Geometry check sheet. Reference: the model listing, model coordinates, mm. Face numbers are marked on the shaded views. Give positions to 0.01 mm unless a question says otherwise; leave off trailing zeros. Loops run counter-clockwise (first coordinate to the right, second up) from the corner with the lowest first, then second, coordinate; pieces in that order, holes last. Notation, with made-up numbers: (8, 1.5) - (42, 1.5) arc R25 cw to (42, 32.5) - close; hole circle Ø11 at (-2, -18.75). An arc over 180 degrees is marked (long way). One line per question, with ' | ' between items. Start each with the question number.
from build123d import *

# Parameters (mm, degrees)
SKETCH1_R             = 5
BOSS_EXTRUDE1_DEPTH   = 24
BOSS_EXTRUDE1_2_DEPTH = 24
BOSS_EXTRUDE1_3_DEPTH = 24
BOSS_EXTRUDE1_4_DEPTH = 24
BOSS_EXTRUDE3_START   = 2
SKETCH1_5_W           = 56.57
SKETCH1_5_H           = 40
SKETCH1_5_R           = 5
BOSS_EXTRUDE3_DEPTH   = 2


with BuildPart() as part:
    # Sketch1 → Boss-Extrude1 (new body)
    with BuildSketch(Plane(origin=(0, 0, 0), x_dir=(1, 0, 0), z_dir=(0, 1, 0))):
        with Locations(Location((-28.285, 5, 0), (0, 0, 270))):
            Circle(SKETCH1_R)
    extrude(amount=-BOSS_EXTRUDE1_DEPTH)



with BuildPart() as body_2:
    # Sketch1 → Boss-Extrude1 2 (new body)
    with BuildSketch(Plane(origin=(0, 0, 0), x_dir=(1, 0, 0), z_dir=(0, 1, 0))):
        with Locations(Location((-28.285, 61.57, 0), (0, 0, 270))):
            Circle(SKETCH1_R)
    extrude(amount=-BOSS_EXTRUDE1_2_DEPTH)


with BuildPart() as body_3:
    # Sketch1 → Boss-Extrude1 3 (new body)
    with BuildSketch(Plane(origin=(0, 0, 0), x_dir=(1, 0, 0), z_dir=(0, 1, 0))):
        with Locations(Location((28.285, 61.57, 0), (0, 0, 270))):
            Circle(SKETCH1_R)
    extrude(amount=-BOSS_EXTRUDE1_3_DEPTH)


with BuildPart() as body_4:
    # Sketch1 → Boss-Extrude1 4 (new body)
    with BuildSketch(Plane(origin=(0, 0, 0), x_dir=(1, 0, 0), z_dir=(0, 1, 0))):
        with Locations(Location((28.285, 5, 0), (0, 0, 270))):
            Circle(SKETCH1_R)
    extrude(amount=-BOSS_EXTRUDE1_4_DEPTH)


with BuildPart() as part_1:
    add(part.part)

    add(body_2.part)  # Boss-Extrude3 merges body 2

    add(body_3.part)  # Boss-Extrude3 merges body 3

    add(body_4.part)  # Boss-Extrude3 merges body 4
    # Sketch1_5 → Boss-Extrude3 (add)
    with BuildSketch(Plane(origin=(0, 0, 0), x_dir=(1, 0, 0), z_dir=(0, 1, 0)).offset(BOSS_EXTRUDE3_START)):
        with BuildLine():
            ThreePointArc((15, 33.285), (0, 18.285), (-15, 33.285))
            Line((-15, 33.285), (-15, 66.57))
            Line((-15, 66.57), (-28.285, 66.57))
            ThreePointArc((-28.285, 66.57), (-24.749466094, 65.105533906), (-23.285, 61.57))
            ThreePointArc((-23.285, 61.57), (-28.285, 56.57), (-33.285, 61.57))
            Line((-33.285, 61.57), (-33.285, 5))
            ThreePointArc((-33.285, 5), (-28.285, 10), (-23.285, 5))
            ThreePointArc((-23.285, 5), (-24.749466094, 1.464466094), (-28.285, 0))
            Line((-28.285, 0), (28.285, 0))
            ThreePointArc((28.285, 0), (24.749466094, 8.535533906), (33.285, 5))
            Line((33.285, 5), (33.285, 61.57))
            ThreePointArc((33.285, 61.57), (24.749466094, 58.034466094), (28.285, 66.57))
            Line((28.285, 66.57), (15, 66.57))
            Line((15, 66.57), (15, 33.285))
        make_face()
        with Locations((0, -20)):
            Rectangle(SKETCH1_5_W, SKETCH1_5_H)
        with Locations(Location((-28.285, 61.57, 0), (0, 0, 90))):
            Circle(SKETCH1_5_R)
        with Locations(Location((28.285, 61.57, 0), (0, 0, 90))):
            Circle(SKETCH1_5_R)
        with Locations(Location((28.285, 5, 0), (0, 0, 270))):
            Circle(SKETCH1_5_R)
        with Locations(Location((-28.285, 5, 0), (0, 0, 270))):
            Circle(SKETCH1_5_R)
    extrude(amount=-BOSS_EXTRUDE3_DEPTH)


solid = part_1.part
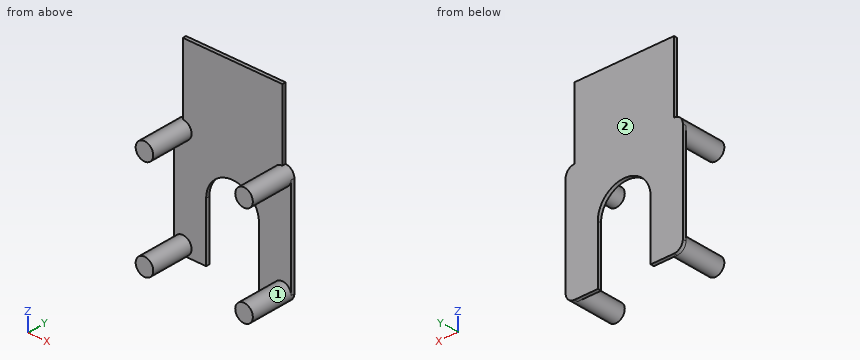
(1) Mould release check, pull along Z, two halves, no side actions. Record for the marked faces 1 and 2: pulls with the +Z half, pulls with the -Z half, needs draft (parallel to the pull), parting line crosses it, or undercut.
(2) Material ranges on line 1 (X direction, y = -15.5, z = -5) (3 decimals); line 2 (Z direction, x = -28, y = -15); line 3 (Y direction, x = 6, z = -4.5), recorded low to high.
(3) Section check C-C, the plane x = -26. Record the boundary of the cut face in (y, z).
(4) Section check A-A, the plane y = -7.5. Record the boundary of the cut face in (x, z) (3 decimals).
(5) Section check B-B, the plane z = -25. Record the boundary of the cut face in (x, y) (3 decimals), and give its area (3 significant figures).
(6) Section check D-D, the plane z = 20. Record the boundary of the cut face in (x, y) (3 decimals).
(7) Depth check by flat-ended pin: pin 1 Ø8 at (x, y) = (12.5, -4.5) entering from -Z; pin 2 Ø3 at (x, z) = (-13, -1.5) entering from -Y; pin 3 Ø1.6 at (y, z) = (1, 15) entering from -X (3 decimals); pin 4 Ø1.6 at (y, z) = (0.5, 10) entering from +X (3 decimals). Enter the tip coordinate at first touch or a pass-through.
Numbers:
1) face 1: undercut | face 2: needs draft
2) line 1: -33.285 to -23.285, 23.285 to 33.285 | line 2: -66.56 to -56.58, -9.99 to -0.01 | line 3: 0 to 2
3) outline: (-24, -66.02) - (0, -66.02) - (0, -66.57) - (2, -66.57) - (2, 40) - (0, 40) - (0, -0.55) - (-24, -0.55) - (-24, -9.45) - (0, -9.45) - (0, -57.12) - (-24, -57.12) - close
4) outline: circle Ø10 at (-28.285, -61.57); circle Ø10 at (-28.285, -5); circle Ø10 at (28.285, -61.57); circle Ø10 at (28.285, -5)
5) outline: (-33.285, 0) - (-12.504, 0) - (-12.504, 2) - (-33.285, 2) - close; (12.504, 0) - (33.285, 0) - (33.285, 2) - (12.504, 2) - close | area: 83.1 mm^2
6) outline: (-28.285, 0) - (28.285, 0) - (28.285, 2) - (-28.285, 2) - close
7) pin 1: through | pin 2: y = 0 | pin 3: x = -28.285 | pin 4: x = 28.285
